from build123d import *

# Parameters (mm, degrees)
EXTRUDE_1_DEPTH     = 3
FILLET_2_R          = 20
SKETCH_2_R          = 2
CUT_EXTRUDE_1_DEPTH = 3
CUT_EXTRUDE_2_DEPTH = 10


with BuildPart() as part:
    # 草图1 → 凸台-拉伸1 (new body)
    with BuildSketch(Plane.XY):
        Polygon((0, 65), (0, 20), (-20, 20), (-20, 0), (200, 0), (200, 20), (180, 20), (180, 65), (150, 65), (150, 123.180584191), (180, 123.180584191), (180, 175), (0, 175), (0, 123.180584191), (30, 123.180584191), (30, 65), align=None)
    extrude(amount=EXTRUDE_1_DEPTH)

    # 圆角2
    fillet_2_edges = [part.edges().sort_by_distance(p)[0] for p in [
        (0, 20, 1.5),
        (180, 20, 1.5),
    ]]
    fillet(fillet_2_edges, radius=FILLET_2_R - 0.0001)  # a hair under: the kernel refuses the full size

    # 草图2 → 切除-拉伸1 (cut)
    with BuildSketch(Plane.XY.offset(3)):
        with Locations((170, 10)):
            Circle(SKETCH_2_R)
        with Locations((190, 10)):
            Circle(SKETCH_2_R)
        with Locations((170, 40)):
            Circle(SKETCH_2_R)
        with Locations((150, 10)):
            Circle(SKETCH_2_R)
        with Locations(Location((30, 10, 0), (0, 0, 180))):
            Circle(SKETCH_2_R)
        with Locations(Location((10, 40, 0), (0, 0, 180))):
            Circle(SKETCH_2_R)
        with Locations(Location((-10, 10, 0), (0, 0, 180))):
            Circle(SKETCH_2_R)
        with Locations(Location((10, 10, 0), (0, 0, 180))):
            Circle(SKETCH_2_R)
        with Locations((170, 145)):
            Circle(SKETCH_2_R)
        with Locations(Location((10, 145, 0), (0, 0, 180))):
            Circle(SKETCH_2_R)
        with Locations((170, 60)):
            Circle(SKETCH_2_R)
        with Locations(Location((10, 60, 0), (0, 0, 180))):
            Circle(SKETCH_2_R)
        with Locations((170, 170)):
            Circle(SKETCH_2_R)
        with Locations(Location((10, 170, 0), (0, 0, 180))):
            Circle(SKETCH_2_R)
    extrude(amount=-CUT_EXTRUDE_1_DEPTH, mode=Mode.SUBTRACT)

    # 草图4 → 切除-拉伸2 (cut)
    with BuildSketch(Plane.XY.offset(3)):
        Polygon((0.5, 175), (0.5, 123.680584191), (30.055288572, 123.680584191), (30, 123.180584191), (-10.698425682, 117.187764406), (-9.272714691, 179.443811016), (-1.573875339, 179.443811016), align=None)
        Polygon((179.5, 175), (179.5, 123.680584191), (149.725032109, 123.680584191), (150, 123.180584191), (194.189444242, 109.302917778), (194.429656629, 189.306403842), (181.700722274, 189.306403842), align=None)
    extrude(amount=-CUT_EXTRUDE_2_DEPTH, mode=Mode.SUBTRACT)


solid = part.part
Verification items for the finished model (mm, model axes). Coordinates: 2 decimals unless noted, no trailing zeros. Order: outer loops, then holes, each group sorted by start corner. A loop starts at its lowest first (then second) coordinate and runs counter-clockwise, first axis right, second up. Notation, with made-up numbers: M -2.5,84.5 L 21.5,84.5 A8 ccw 21.5,88.5 Z; hole C 68,75.5 d7. An arc over 180 degrees is marked long. One line per item, written item: value. Start each with the question number.
Item 1: Scan lines: probe 1 along X at (y, z) = (145, 1.7); probe 2 along Y at (x, z) = (2, 0.3); probe 3 along X at (y, z) = (81, 2.35). Record each from-to range of solid material in increasing order.
Item 2: Gauge pin test, flat ends, axial feed: pin 1 (0.9 mm diameter, centred on y = 94.5, z = 1.5, fed in from +X); pin 2 (0.9 mm diameter, centred on y = 162, z = 2, fed in from -X); pin 3 (0.9 mm diameter, centred on y = 150.5, z = 1, fed in from +X). Record the tip position at first contact, or that the pin passes through.
Item 3: Sectioned sample at C-C (y = 162). Enter the section's corners in (x, z), then the cut area to 3 significant figures.
Item 4: Sectioned sample at B-B (x = -5). Enter the section's corners in (y, z), then the cut area to 3 significant figures.
Item 5: Sectioned sample at A-A (z = 0.9). Count the separate pieces of the cut face and the enclosed holes in it, then the cut area to 3 significant figures.
Conclusion:
1. probe 1: x = 0.5 to 8, 12 to 168, 172 to 179.5
1. probe 2: y = 0 to 65, 123.68 to 175
1. probe 3: x = 30 to 150
2. pin 1: stops at x = 150
2. pin 2: stops at x = 0.5
2. pin 3: stops at x = 179.5
3. outline: M 0.5,0 L 179.5,0 L 179.5,3 L 0.5,3 Z
3. area: 537 mm^2
4. outline: M 0,0 L 26.77,0 L 26.77,3 L 0,3 Z
4. area: 80.3 mm^2
5. separate pieces: 1
5. enclosed holes: 14
5. area: 28,700 mm^2
